Part model, mm, in its own coordinate system. A direction names the side the tool comes from. Coordinates: 2 decimals unless noted, no trailing zeros. Loops run counter-clockwise (first coordinate to the right, second up) from the corner with the lowest first, then second, coordinate; pieces in that order, holes last. Notation, with made-up numbers: M -21,53 L 7,53 A8 cw 7,62 Z; hole C -17,10 d9. An arc over 180 degrees is marked long. Use a Markdown table: item, result. Add a question column.
1) Tool access for faces 1 (the cylindrical face through (14.857, 9.483, -1.615)), 2 (the cylindrical face through (-67.906, 5.635, -21.717)), 3 (the cylindrical face through (-104.7, 6.06, -57.84)): list every direction of +Z, -Z, +X, -X, +Y, -Y with a clear straight run to the whole face (end or side of a thin tool).
2) Wall check: probe 1 along X at (y, z) = (-2.85, 57.15) (3 decimals); probe 2 along Y at (x, z) = (-5, 0); probe 3 along Z at (x, y) = (-44.45, 2.5). Give the ranges that are in metal, low to high. Write a range as from..to.
3) Pull direction Z, two halves, no side cores. Call faces 4 (the flat face through (-74, -5.08, 43)), 5 (the flat face through (-45, 6, -63.5)), 6 (the cylindrical face through (-90.942, -2.504, 10.324)): released by +Z, released by -Z, zero draft, split by the parting line, or undercut.
4) Pin check, flat tips, straight feed: pin 1 Ø13.5 at (x, z) = (-44.45, 0) entering from -Y; pin 2 Ø23 at (x, z) = (-44.45, 0) entering from -Y. Stop position of each tip, or through.
5) Band-saw the part on A-A (z = 57.15). List the corners of the cut face in (x, y) (3 decimals).
from build123d import *

# Parameters (mm, degrees)
SKETCH5_W                = 127
SKETCH5_H                = 127
SKETCH5_R                = 38.1
SKETCH5_R_2              = 3.175
BOSS_EXTRUDE2_DEPTH      = 17.50822
CUT_EXTRUDE5_REACH       = 145.066
SKETCH8_R                = 3.175
CUT_EXTRUDE9_REACH       = 169.597
SKETCH10_R               = 0.79375
SKETCH11_W               = 127
SKETCH11_H               = 127
SKETCH11_R               = 47.625
BOSS_EXTRUDE3_DEPTH      = 5.08
SKETCH12_R               = 26.9875
SKETCH12_R_2             = 23.8125
CUT_EXTRUDE10_DEPTH      = 2.159
CUT_EXTRUDE12_DEPTH      = 128.262249687
CUT_EXTRUDE12_DEPTH_BACK = 128.262249687
SKETCH14_R               = 3.175
SKETCH15_R               = 19.05
CUT_EXTRUDE13_DEPTH      = 2.032
CIRPATTERN1_COUNT        = 9
CHAMFER1_SIZE            = 0.508


# Read off the part's stored shape, not the designer's step: Q (0.332) Diameter Hole1
with BuildPart() as part:
    # Sketch1 → Revolve1 (revolve)
    with BuildSketch(Plane.XY, mode=Mode.PRIVATE) as revolve1_sk:
        with BuildLine():
            Line((-38.49624, 17.50822), (0, 17.50822))
            Line((0, 17.50822), (0, 0))
            Line((0, 0), (-33.4645, 0))
            Line((-33.4645, 0), (-33.4645, 3.456354569))
            ThreePointArc((-33.4645, 3.456354569), (-33.872854569, 4.980354569), (-34.9885, 6.096))
            Line((-34.9885, 6.096), (-38.49624, 8.96874))
            Line((-38.49624, 8.96874), (-38.49624, 17.50822))
        make_face()
    revolve(revolve1_sk.sketch.rotate(Axis((-44.45, 101.60464546, 0), (0, 1, 0)), 90), axis=Axis((-44.45, 101.60464546, 0), (0, 1, 0)))

    # Sketch5 → Boss-Extrude2 (add)
    with BuildSketch(Plane.XZ):
        with Locations((-44.45, 0)):
            Rectangle(SKETCH5_W, SKETCH5_H)
        with Locations((-44.45, 0)):
            Circle(SKETCH5_R, mode=Mode.SUBTRACT)
        with Locations(Location((-101.6, 57.15, 0), (0, 0, 270))):
            Circle(SKETCH5_R_2, mode=Mode.SUBTRACT)
        with Locations(Location((12.7, 57.15, 0), (0, 0, 90))):
            Circle(SKETCH5_R_2, mode=Mode.SUBTRACT)
        with Locations(Location((12.7, -57.15, 0), (0, 0, 270))):
            Circle(SKETCH5_R_2, mode=Mode.SUBTRACT)
        with Locations(Location((-101.6, -57.15, 0), (0, 0, 90))):
            Circle(SKETCH5_R_2, mode=Mode.SUBTRACT)
    extrude(amount=-BOSS_EXTRUDE2_DEPTH)

    # Sketch8 → Cut-Extrude5 (cut, up to next)
    with BuildSketch(Plane(origin=(19.05, 0, 0), x_dir=(0, 0, -1), z_dir=(1, 0, 0)), mode=Mode.PRIVATE) as cut_extrude5_sk1:
        with Locations((0, 5.588)):
            Circle(SKETCH8_R)
    cut_extrude5_tool1 = extrude(cut_extrude5_sk1.sketch, amount=-CUT_EXTRUDE5_REACH, mode=Mode.PRIVATE) & part.part
    add(cut_extrude5_tool1.solids().sort_by_distance((19.05, 5.588, 0))[0], mode=Mode.SUBTRACT)

    # Sketch10 → Cut-Extrude9 (cut, up to next)
    with BuildSketch(Plane.XY.offset(63.5), mode=Mode.PRIVATE) as cut_extrude9_sk1:
        with Locations((-39.37, 5.588)):
            Circle(SKETCH10_R)
    cut_extrude9_tool1 = extrude(cut_extrude9_sk1.sketch, amount=-CUT_EXTRUDE9_REACH, mode=Mode.PRIVATE) & part.part
    add(cut_extrude9_tool1.solids().sort_by_distance((-39.37, 5.588, 63.5))[0], mode=Mode.SUBTRACT)

    # Sketch11 → Boss-Extrude3 (add)
    with BuildSketch(Plane.XZ):
        with Locations((-44.45, 0)):
            Rectangle(SKETCH11_W, SKETCH11_H)
        with Locations(Location((-44.45, 0, 0), (0, 0, 270))):
            Circle(SKETCH11_R, mode=Mode.SUBTRACT)
    extrude(amount=BOSS_EXTRUDE3_DEPTH)

    # Sketch12 → Cut-Extrude10 (cut)
    with BuildSketch(Plane.XZ):
        with Locations(Location((-44.45, 0, 0), (0, 0, 270))):
            Circle(SKETCH12_R)
        with Locations(Location((-44.45, 0, 0), (0, 0, 270))):
            Circle(SKETCH12_R_2, mode=Mode.SUBTRACT)
    extrude(amount=-CUT_EXTRUDE10_DEPTH, mode=Mode.SUBTRACT)

    # Sketch14 → Cut-Extrude12 (cut, two sides: drawn at the far end of the back side and taken through both)
    with BuildSketch(Plane(origin=(0, 17.50822, 0), x_dir=(1, 0, 0), z_dir=(0, 1, 0)).offset(-CUT_EXTRUDE12_DEPTH_BACK)):
        with Locations(Location((-101.6, 57.15, 0), (0, 0, 270))):
            Circle(SKETCH14_R)
        with Locations(Location((12.7, 57.15, 0), (0, 0, 270))):
            Circle(SKETCH14_R)
        with Locations(Location((12.7, -57.15, 0), (0, 0, 270))):
            Circle(SKETCH14_R)
        with Locations(Location((-101.6, -57.15, 0), (0, 0, 270))):
            Circle(SKETCH14_R)
    extrude(amount=CUT_EXTRUDE12_DEPTH + CUT_EXTRUDE12_DEPTH_BACK, mode=Mode.SUBTRACT)

    # Sketch15 → Cut-Extrude13 (cut)
    with BuildSketch(Plane.XZ):
        with Locations(Location((-44.45, 0, 0), (0, 0, 270))):
            Circle(SKETCH15_R)
    extrude(amount=-CUT_EXTRUDE13_DEPTH, mode=Mode.SUBTRACT)

    # Sketch19 → Tapped Hole for 1/4-20 Helicoil2 (revolve, cut)
    with BuildSketch(Plane(origin=(-79.375, 0, 0), x_dir=(0, 0, -1), z_dir=(1, 0, 0))):
        Polygon((0, 0), (0, 13.459827343), (3.3782, 11.43), (3.3782, 0), align=None)
    tapped_hole_for_1_4_20_helicoil2 = revolve(axis=Axis((-79.375, -6.35, 0), (0, 1, 0)), mode=Mode.SUBTRACT)

    # CirPattern1: Tapped Hole for 1/4-20 Helicoil2 ×9 about axis
    cirpattern1_axis = Axis((-44.45, 0, 0), (0, 1, 0))
    for i in range(1, CIRPATTERN1_COUNT):
        add(tapped_hole_for_1_4_20_helicoil2.rotate(cirpattern1_axis, i * 360 / CIRPATTERN1_COUNT), mode=Mode.SUBTRACT)

    # Chamfer1
    chamfer1_edges = [part.edges().sort_by_distance(p)[0] for p in [
        (-44.45, 0, 19.05),
    ]]
    chamfer(chamfer1_edges, length=CHAMFER1_SIZE)

    # Q (0.332) Diameter Hole1 outline → Q (0.332) Diameter Hole1 (revolve, cut)
    with BuildSketch(Plane(origin=(-39.37, 5.588, 0), x_dir=(1, 0, 0), z_dir=(0, -1, 0))):
        Polygon((0.79375, 63.5), (0.79375, 53.315464402), (4.2164, 55.372), (4.2164, 63.133382579), (4.8514, 63.5), align=None)
    revolve(axis=Axis((-39.37, 5.588, 0), (0, 0, 1)), mode=Mode.SUBTRACT)

    # Q _0.332_ Diameter Hole1 2 outline → Q _0.332_ Diameter Hole1 2 (revolve, cut)
    with BuildSketch(Plane(origin=(0, 5.588, 0), x_dir=(0, 1, 0), z_dir=(0, 0, -1))):
        Polygon((3.175, 19.05), (3.175, 10.296263751), (4.2164, 10.922), (4.2164, 18.683382579), (4.8514, 19.05), align=None)
    revolve(axis=Axis((0, 5.588, 0), (1, 0, 0)), mode=Mode.SUBTRACT)


solid = part.part
Entries:
| question | item | result |
|---|---|---|
| 1 | face 1 | +X |
| 1 | face 2 | -Y |
| 1 | face 3 | +Y, -Y |
| 2 | probe 1 | -107.95..-104.775, -98.425..9.525, 15.875..19.05 |
| 2 | probe 2 | 0..2.41, 8.76..17.51 |
| 2 | probe 3 | -63.5..-10.99, 10.99..63.5 |
| 3 | face 4 | zero draft |
| 3 | face 5 | released by -Z |
| 3 | face 6 | undercut |
| 4 | pin 1 | y = 8.32 |
| 4 | pin 2 | y = 2.03 |
| 5 | outline | M -107.95,-5.08 L -104.775,-5.08 L -104.775,17.508 L -107.95,17.508 Z; M -98.425,-5.08 L 9.525,-5.08 L 9.525,17.508 L -98.425,17.508 Z; M 15.875,-5.08 L 19.05,-5.08 L 19.05,17.508 L 15.875,17.508 Z; hole C -39.37,5.588 d8.433 |
